from build123d import *

# Parameters (mm, degrees)
SZKIC1_W                    = 95
SZKIC1_H                    = 60
DODANIE_WYCI_GNI_CIE1_DEPTH = 20
KONWERTUJ_BRY_1_DEPTH       = 60


# Read off the part's stored shape, not the designer's step: Konwertuj bryłę1
with BuildPart() as part:
    # Szkic1 → Dodanie-wyciągnięcie1 (new body)
    with BuildSketch(Plane.XY):
        with Locations((47.5, 30)):
            Rectangle(SZKIC1_W, SZKIC1_H)
    extrude(amount=DODANIE_WYCI_GNI_CIE1_DEPTH)

    # Konwertuj bryłę1 outline → Konwertuj bryłę1 (cut)
    with BuildSketch(Plane(origin=(0, 0, 0), x_dir=(1, 0, 0), z_dir=(0, 1, 0))):
        with BuildLine():
            Line((95, 0), (91, 0))
            ThreePointArc((91, 0), (93.828427125, -1.171572875), (95, -4))
            Line((95, -4), (95, 0))
        make_face()
        with BuildLine():
            ThreePointArc((0, -4), (1.171572875, -1.171572875), (4, 0))
            Line((4, 0), (0, 0))
            Line((0, 0), (0, -4))
        make_face()
        with BuildLine():
            Line((2, -20), (93, -20))
            Line((93, -20), (93, -4))
            ThreePointArc((93, -4), (92.414213562, -2.585786438), (91, -2))
            Line((91, -2), (4, -2))
            ThreePointArc((4, -2), (2.585786438, -2.585786438), (2, -4))
            Line((2, -4), (2, -20))
        make_face()
    extrude(amount=KONWERTUJ_BRY_1_DEPTH, mode=Mode.SUBTRACT)


solid = part.part
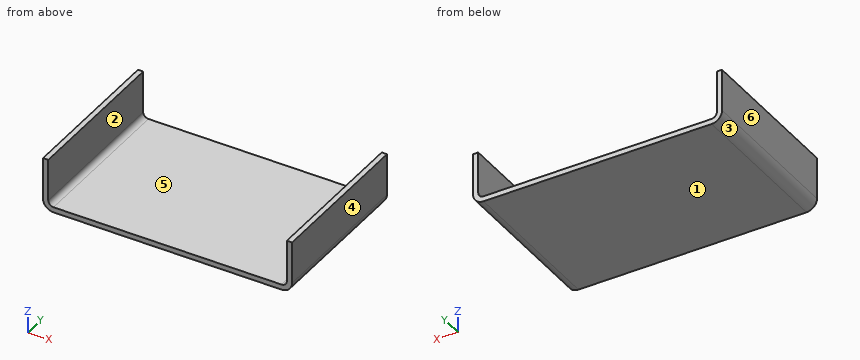
The model under review builds one solid part; all positions refer to its coordinate system, in mm. Face numbers are marked on the shaded views. A direction names the side the tool comes from. Round coordinates to 2 decimals unless told otherwise and drop trailing zeros. Loops run counter-clockwise (first coordinate to the right, second up) from the corner with the lowest first, then second, coordinate; pieces in that order, holes last. Notation, with made-up numbers: (-1.75, -2.75) -> (25.25, -2.75) arc R25 cw to (25.25, 10.25) -> close; hole circle Ø4 at (32.5, 73). An arc over 180 degrees is marked (long way). Write item = value, one per line. Start each with the question number.
Item 1: Insertion check: pin 1 (1 mm diameter, centred on x = 36.5, y = 43.5, fed in from +Z); pin 2 (1 mm diameter, centred on y = 32.5, z = 2, fed in from +X). Each pin has a flat end and moves straight along its axis. Give the tip position at first contact, or say it passes through.
Item 2: Take a section at A-A on z = 18.75. Give the boundary of the cut face in (x, y).
Item 3: To check wall thickness, follow L1, parallel to X at y = 36, z = 5.5; L2, parallel to Z at x = 7.5, y = 35; L3, parallel to X at y = 43, z = 2.75. State the ranges of each line that lie inside material, in increasing order.
Item 4: Take a section at B-B on y = 4. Give the boundary of the cut face in (x, z).
Item 5: For the marked faces 5 and 6, list the 3-axis set-ups (+Z, -Z, +X, -X, +Y, -Y) from which the entire face can be reached by the end or side of a thin tool; tool diameter is ignored.
Item 6: Mouldability with a two-part tool opening along X and no side actions: class the marked faces 1, 2, 3 and 4 as released by +X, released by -X, zero draft, split by the parting line, or undercut.
Item 7: Take a section at C-C on x = 85.5. Give the boundary of the cut face in (y, z), plus the area to 3 significant figures.
Result:
q1.pin_1 = 2
q1.pin_2 = 94.71
q2.outline = (0, 0) -> (2, 0) -> (2, 60) -> (0, 60) -> close; (93, 0) -> (95, 0) -> (95, 60) -> (93, 60) -> close
q3.L1 = 0 to 2, 93 to 95
q3.L2 = 0 to 2
q3.L3 = 0.2 to 2.44, 92.56 to 94.8
q4.outline = (0, 4) arc R4 ccw to (4, 0) -> (91, 0) arc R4 ccw to (95, 4) -> (95, 20) -> (93, 20) -> (93, 4) arc R2 cw to (91, 2) -> (4, 2) arc R2 cw to (2, 4) -> (2, 20) -> (0, 20) -> close
q5.face_5 = +Z, +Y, -Y
q5.face_6 = +Z, -Z, -X, +Y, -Y
q6.face_1 = zero draft
q6.face_2 = undercut
q6.face_3 = released by -X
q6.face_4 = released by +X
q7.outline = (0, 0) -> (60, 0) -> (60, 2) -> (0, 2) -> close
q7.area = 120 mm²
